CAD build for the part. Positions are in the model's coordinates, mm. A direction names the side the tool comes from. Round coordinates to 2 decimals unless told otherwise and drop trailing zeros. Write each loop counter-clockwise with the first axis right and the second up, starting at its lowest first coordinate (ties: lowest second). Pieces come first, ordered by that corner, then holes. Notation, with made-up numbers: (-33.75, 61) - (13.25, 61) arc R16 cw to (13.25, 71) - close; hole circle Ø2 at (22.25, -33.5). An arc over 180 degrees is marked (long way). Use one line per item in the form item = value. Start each with the question number.
Item 1: Drill centre lines: L1, parallel to X at y = 15, z = 0; L2, parallel to X at y = 22, z = 9; L3, parallel to X at y = 20.5, z = -37. Where is each one in solid material? Low to high.
Item 2: Tool access for faces 1 (the cylindrical face through (1.19, 24.65, 37.48)), 2 (the flat face through (17.92, 24.65, -86.41)): list every direction of +Z, -Z, +X, -X, +Y, -Y with a clear straight run to the whole face (end or side of a thin tool).
Item 3: Pull direction Z, two halves, no side cores. Call faces 3 (the cylindrical face through (25.253, 24.65, -43.797)), 4 (the flat face through (-35, 25, -96.546)), 5 (the flat face through (-40, 25, -76)): +Z half, -Z half, draft (parallel to the pull), parting line (faces both ways), or undercut.
Item 4: Pin check, flat tips, straight feed: pin 1 (3 mm diameter, centred on x = 23, y = 10, fed in from -Z); pin 2 (6 mm diameter, centred on x = -18.5, y = 26, fed in from +Z); pin 3 (3 mm diameter, centred on y = 15, z = -2.5, fed in from -X). Stop position of each tip, or through.
Item 5: Band-saw the part on C-C, the plane y = 17. List the corners of the cut face in (x, z), and give its area (3 significant figures).
Item 6: Band-saw the part on B-B, the plane z = 2.5. List the corners of the cut face in (x, y), and give its area (3 significant figures).
Item 7: Band-saw the part on A-A, the plane x = 0. List the corners of the cut face in (y, z).
from build123d import *

# Parameters (mm, degrees)
CROQUIS2_R              = 22.5
SALIENTE_EXTRUIR1_DEPTH = 50


with BuildPart() as part:
    # Croquis2 → Saliente-Extruir1 (new body)
    with BuildSketch(Plane(origin=(0, 0, 0), x_dir=(1, 0, 0), z_dir=(0, 1, 0))):
        with BuildLine():
            Line((-6.164928148, 76.54643814), (6.164928148, 76.54643814))
            Line((6.164928148, 76.54643814), (30, 96.54643814))
            Line((30, 96.54643814), (40, 96.54643814))
            Line((40, 96.54643814), (40, 56.54643814))
            ThreePointArc((40, 56.54643814), (25.155667723, 43.525085879), (28.726666617, 24.104535363))
            ThreePointArc((28.726666617, 24.104535363), (0, -37.5), (-28.726666617, 24.104535363))
            ThreePointArc((-28.726666617, 24.104535363), (-25.155667723, 43.525085879), (-40, 56.54643814))
            Line((-40, 56.54643814), (-40, 96.54643814))
            Line((-40, 96.54643814), (-30, 96.54643814))
            Line((-30, 96.54643814), (-6.164928148, 76.54643814))
        make_face()
        Circle(CROQUIS2_R, mode=Mode.SUBTRACT)
    extrude(amount=SALIENTE_EXTRUIR1_DEPTH)


solid = part.part
Determined:
q1.L1 = -37.5 to -22.5, 22.5 to 37.5
q1.L2 = -36.4 to -20.62, 20.62 to 36.4
q1.L3 = -24.05 to 24.05
q2.face_1 = +Y, -Y
q2.face_2 = -Z, +Y, -Y
q3.face_3 = undercut
q3.face_4 = -Z half
q3.face_5 = draft
q4.pin_1 = -91.93
q4.pin_2 = 34.15
q4.pin_3 = -37.49
q5.outline = (-40, -96.55) - (-30, -96.55) - (-6.16, -76.55) - (6.16, -76.55) - (30, -96.55) - (40, -96.55) - (40, -56.55) arc R20 cw to (28.73, -24.1) arc R37.5 ccw (long way) to (-28.73, -24.1) arc R20 cw to (-40, -56.55) - close; hole circle Ø45 at (0, 0)
q5.area = 6,530 mm²
q6.outline = (-37.42, 0) - (-22.36, 0) - (-22.36, 50) - (-37.42, 50) - close; (22.36, 0) - (37.42, 0) - (37.42, 50) - (22.36, 50) - close
q6.area = 1,510 mm²
q7.outline = (0, -76.55) - (50, -76.55) - (50, -22.5) - (0, -22.5) - close; (0, 22.5) - (50, 22.5) - (50, 37.5) - (0, 37.5) - close
